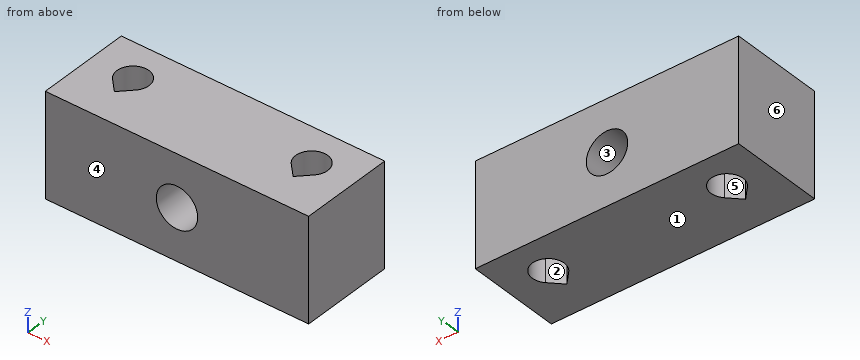
from build123d import *

# Parameters (mm, degrees)
SKETCH1_W           = 28
SKETCH1_H           = 11
BOSS_EXTRUDE1_DEPTH = 10
CUT_EXTRUDE1_DEPTH  = 62.911246959
CUT_EXTRUDE2_DEPTH  = 62.911246959
HOLE1_D             = 4.4


with BuildPart() as part:
    # Sketch1 → Boss-Extrude1 (new body)
    with BuildSketch(Plane.XZ.offset(46)):
        with Locations((25.95, 5.5)):
            Rectangle(SKETCH1_W, SKETCH1_H)
    extrude(amount=-BOSS_EXTRUDE1_DEPTH)

    # Sketch2 → Cut-Extrude1 (cut, through all)
    with BuildSketch(Plane.XY.offset(11)):
        with BuildLine():
            Line((35.425, -42.447246117), (36.647877661, -41.18091923))
            ThreePointArc((36.647877661, -41.18091923), (35.425, -38.3), (34.202122339, -41.18091923))
            Line((34.202122339, -41.18091923), (35.425, -42.447246117))
        make_face()
    extrude(amount=-CUT_EXTRUDE1_DEPTH, mode=Mode.SUBTRACT)

    # Sketch3 → Cut-Extrude2 (cut, through all)
    with BuildSketch(Plane(origin=(0, 0, 0), x_dir=(-1, 0, 0), z_dir=(0, 0, -1))):
        with BuildLine():
            Line((-17.647877661, -41.18091923), (-16.425, -42.447246117))
            Line((-16.425, -42.447246117), (-15.202122339, -41.18091923))
            ThreePointArc((-15.202122339, -41.18091923), (-16.425, -38.3), (-17.647877661, -41.18091923))
        make_face()
    extrude(amount=-CUT_EXTRUDE2_DEPTH, mode=Mode.SUBTRACT)

    # Hole1 (through all)
    with Locations(Plane.XZ.offset(46)):
        with Locations((25.95, 5.5)):
            Hole(HOLE1_D / 2)


solid = part.part
Could you check a few things on this model? Use its own coordinates, in mm. Face numbers are marked on the shaded views. A direction names the side the tool comes from. Coordinates: 2 decimals unless noted, no trailing zeros. Loops run counter-clockwise (first coordinate to the right, second up) from the corner with the lowest first, then second, coordinate; pieces in that order, holes last.
1. For the marked faces 1 and 2, which set-ups out of +Z, -Z, +X, -X, +Y, -Y let a thin tool reach every point of the face, with its end or its side?
2. Imagine slicing it at C-C (x = 25.95). Please give me the cut outline in (y, z), and give its area (3 significant figures).
3. We'd pull the mould along X, two halves only. Please class the marked faces 3, 4, 5 and 6: released by +X, released by -X, zero draft, split by the parting line, or undercut.
4. I need wall thicknesses on L1, parallel to X at y = -40, z = 2.75 (3 decimals); L2, parallel to Z at x = 25.95, y = -42; L3, parallel to X at y = -40, z = 5 (3 decimals). Which ranges of each line are inside material? Lowest first, please.
5. Imagine slicing it at B-B (z = 5.5). Please give me the cut outline in (x, y) (3 decimals), and give its area (3 significant figures).
6. Imagine slicing it at A-A (y = -40). Please give me the cut outline in (x, z) (3 decimals).
7. Imagine slicing it at D-D (z = 8.25). Please give me the cut outline in (x, y) (3 decimals).
Computed values:
1. face 1: -Z, +X, -X, +Y, -Y
1. face 2: +Z, -Z
2. outline: (-46, 0) - (-36, 0) - (-36, 3.3) - (-46, 3.3) - close; (-46, 7.7) - (-36, 7.7) - (-36, 11) - (-46, 11) - close
2. area: 66.0 mm2
3. face 3: undercut
3. face 4: zero draft
3. face 5: undercut
3. face 6: released by -X
4. L1: x = 11.95 to 14.725, 18.125 to 33.725, 37.125 to 39.95
4. L2: z = 0 to 3.3, 7.7 to 11
4. L3: x = 11.95 to 14.725, 18.125 to 23.808, 28.092 to 33.725, 37.125 to 39.95
5. outline: (11.95, -46) - (23.75, -46) - (23.75, -36) - (11.95, -36) - close; (28.15, -46) - (39.95, -46) - (39.95, -36) - (28.15, -36) - close; hole (15.202, -41.181) - (16.425, -42.447) - (17.648, -41.181) arc R1.7 ccw (long way) to start; hole (34.202, -41.181) - (35.425, -42.447) - (36.648, -41.181) arc R1.7 ccw (long way) to start
5. area: 216 mm2
6. outline: (11.95, 0) - (14.725, 0) - (14.725, 11) - (11.95, 11) - close; (18.125, 0) - (33.725, 0) - (33.725, 11) - (18.125, 11) - close; (37.125, 0) - (39.95, 0) - (39.95, 11) - (37.125, 11) - close; hole circle Ø4.4 at (25.95, 5.5)
7. outline: (11.95, -46) - (39.95, -46) - (39.95, -36) - (11.95, -36) - close; hole (15.202, -41.181) - (16.425, -42.447) - (17.648, -41.181) arc R1.7 ccw (long way) to start; hole (34.202, -41.181) - (35.425, -42.447) - (36.648, -41.181) arc R1.7 ccw (long way) to start
